```python
from build123d import *

# Parameters (mm, degrees)
F0_W        = 36.83
F0_H        = 2.54
F1_DEPTH    = 7.62
F3_T1_DEPTH = 58.8270452561
F4_DEPTH    = 25.4


# Not quite as in the source:
# - a fillet or chamfer that OpenCascade refuses, or shapes differently, is made with other operations: its cross-section is extruded or revolved along the edge and cut away or added


with BuildPart() as f1:
    # F0 (on Top) → F1 (new body)
    with BuildSketch(Plane.XY):
        with Locations((-0.635, 1.27)):
            Rectangle(F0_W, F0_H)
    extrude(amount=F1_DEPTH)

    # F3: fillet of radius 5.08 on 1 edges, made by hand

    # F3_s2 → F3_t1 (cut)
    with BuildSketch(Plane.YZ.offset(-30.0485226281)):
        with BuildLine():
            ThreePointArc((2.54, 3.2205909488), (1.8594090512, 5.7605909488), (0, 7.62))
            Line((0, 7.62), (2.54, 7.62))
            Line((2.54, 7.62), (2.54, 3.2205909488))
        make_face()
    extrude(amount=F3_T1_DEPTH, mode=Mode.SUBTRACT)

    # F2 (on face) → F4 (cut)
    with BuildSketch(Plane.XZ):
        Polygon((-15.875, 6.1822954744), (-15.0449409051, 7.62), (-16.7050590949, 7.62), align=None)
        Polygon((-4.7382939367, 7.62), (-6.6917060633, 7.62), (-5.715, 5.9282954744), align=None)
        Polygon((5.2750590949, 7.62), (3.6149409051, 7.62), (4.445, 6.1822954744), align=None)
        Polygon((15.4350590949, 7.62), (13.7749409051, 7.62), (14.605, 6.1822954744), align=None)
    extrude(amount=-F4_DEPTH, mode=Mode.SUBTRACT)


solid = f1.part
```
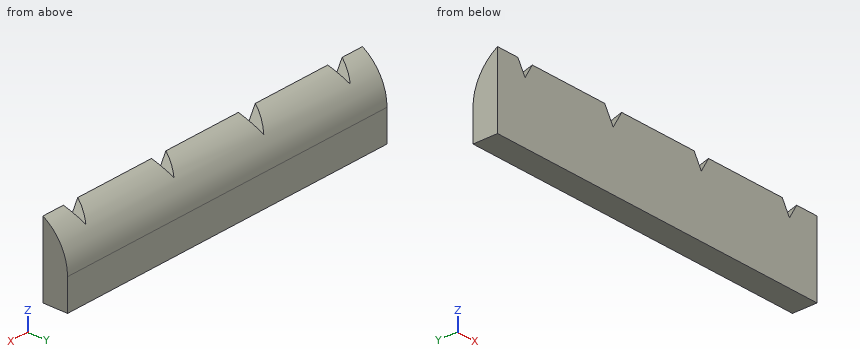
Geometry check sheet. Reference: the model listing, model coordinates, mm. Coordinates: 2 decimals unless noted, no trailing zeros. Loops run counter-clockwise (first coordinate to the right, second up) from the corner with the lowest first, then second, coordinate; pieces in that order, holes last. Notation, with made-up numbers: (-22, 38) -> (15, 38) arc R23 ccw to (15, 52) -> close; hole circle Ø2 at (17.5, -34.5). An arc over 180 degrees is marked (long way). Put each result on its own line as item: value.
1) Cross-section at C-C on x = 10. Record the boundary of the cut face in (y, z).
Result set:
outline: (0, 0) -> (2.54, 0) -> (2.54, 3.22) arc R5.08 ccw to (0, 7.62) -> close
2) Thickness scan on line 1 (Y direction, x = 12, z = 3.5); line 2 (Z direction, x = 4, y = 1.3); line 3 (Y direction, x = 12.5, z = 5). Record the ranges inside material, lowest first.
Result set:
line 1: y = 0 to 2.53
line 2: z = 0 to 6.55
line 3: y = 0 to 2.22
3) Cross-section at D-D on z = 5.5. Record the boundary of the cut face in (x, y).
Result set:
outline: (-19.05, 0) -> (17.78, 0) -> (17.78, 2) -> (-19.05, 2) -> close
4) Cross-section at A-A on z = 7. Record the boundary of the cut face in (x, y).
Result set:
outline: (-19.05, 0) -> (-16.35, 0) -> (-16.35, 0.85) -> (-19.05, 0.85) -> close; (-15.4, 0) -> (-6.33, 0) -> (-6.33, 0.85) -> (-15.4, 0.85) -> close; (-5.1, 0) -> (3.97, 0) -> (3.97, 0.85) -> (-5.1, 0.85) -> close; (4.92, 0) -> (14.13, 0) -> (14.13, 0.85) -> (4.92, 0.85) -> close; (15.08, 0) -> (17.78, 0) -> (17.78, 0.85) -> (15.08, 0.85) -> close
5) Cross-section at B-B on y = 0.35. Record the boundary of the cut face in (x, z) (3 decimals), plus the area to 3 significant figures.
Result set:
outline: (-19.05, 0) -> (17.78, 0) -> (17.78, 7.398) -> (15.307, 7.398) -> (14.605, 6.182) -> (13.903, 7.398) -> (5.147, 7.398) -> (4.445, 6.182) -> (3.743, 7.398) -> (-4.866, 7.398) -> (-5.715, 5.928) -> (-6.564, 7.398) -> (-15.173, 7.398) -> (-15.875, 6.182) -> (-16.577, 7.398) -> (-19.05, 7.398) -> close
area: 269 mm^2
6) Gauge pin test, flat end, axial feed: pin 1 Ø2 at (x, z) = (12, 5) entering from +Y. Record the tip position at first contact, or that the pin passes through.
Result set:
pin 1: stops at y = 2.48
